from build123d import *

# Parameters (mm, degrees)
SKETCH_1_W          = 390
SKETCH_1_H          = 70
EXTRUDE_1_DEPTH     = 90
SKETCH_2_W          = 20
SKETCH_2_H          = 20
CUT_EXTRUDE_1_DEPTH = 85
CUT_EXTRUDE_2_DEPTH = 20
CUT_EXTRUDE_3_DEPTH = 20
CUT_EXTRUDE_4_DEPTH = 86.5


with BuildPart() as part:
    # 草圖1 → 填料-伸長1 (new body)
    with BuildSketch(Plane(origin=(0, 0, 0), x_dir=(1, 0, 0), z_dir=(0, 1, 0))):
        Rectangle(SKETCH_1_W, SKETCH_1_H)
    extrude(amount=EXTRUDE_1_DEPTH)

    # 草圖2 → 除料-伸長1 (cut)
    with BuildSketch(Plane.XY.offset(35)):
        with Locations((185, 10)):
            Rectangle(SKETCH_2_W, SKETCH_2_H)
        with Locations((-185, 10)):
            Rectangle(SKETCH_2_W, SKETCH_2_H)
    extrude(amount=-CUT_EXTRUDE_1_DEPTH, mode=Mode.SUBTRACT)

    # 草圖3 → 除料-伸長2 (cut)
    with BuildSketch(Plane(origin=(195, 0, 0), x_dir=(0, 0, -1), z_dir=(1, 0, 0))):
        Polygon((35, 20), (11.5, 20), (35, 43.5), align=None)
    cut_extrude_2 = extrude(amount=-CUT_EXTRUDE_2_DEPTH, mode=Mode.SUBTRACT)

    # 鏡射1: 除料-伸長2 across plane
    add(cut_extrude_2.mirror(Plane(origin=(0, 0, 0), x_dir=(0, 0, 1), z_dir=(1, 0, 0))), mode=Mode.SUBTRACT)

    # 草圖4 → 除料-伸長3 (cut)
    with BuildSketch(Plane.XZ):
        Polygon((-151.5, -35), (-175, -35), (-175, -11.5), align=None)
        Polygon((175, -11.5), (151.5, -35), (175, -35), align=None)
    extrude(amount=-CUT_EXTRUDE_3_DEPTH, mode=Mode.SUBTRACT)

    # 草圖5 → 除料-伸長4 (cut)
    with BuildSketch(Plane(origin=(0, 90, 0), x_dir=(1, 0, 0), z_dir=(0, 1, 0))):
        Polygon((-171.5, 10.050252532), (-171.5, -31.5), (171.5, -31.5), (171.5, 10.050252532), (150.050252532, 31.5), (-150.050252532, 31.5), align=None)
    extrude(amount=-CUT_EXTRUDE_4_DEPTH, mode=Mode.SUBTRACT)


solid = part.part
Verification items for the finished model (mm, model axes). A direction names the side the tool comes from. Coordinates: 2 decimals unless noted, no trailing zeros. Order: outer loops, then holes, each group sorted by start corner. A loop starts at its lowest first (then second) coordinate and runs counter-clockwise, first axis right, second up.
Item 1: Section check D-D, the plane y = 48.5. Enter the section's corners in (x, z), then the cut area to 3 significant figures.
Filled in:
outline: (-195, -35) - (195, -35) - (195, 35) - (-195, 35) - close; hole (-171.5, -10.05) - (-150.05, -31.5) - (150.05, -31.5) - (171.5, -10.05) - (171.5, 31.5) - (-171.5, 31.5) - close
area: 6,150 mm2
Item 2: Section check C-C, the plane x = 134. Enter the section's corners in (y, z), then the cut area to 4 significant figures.
Filled in:
outline: (0, -35) - (90, -35) - (90, -31.5) - (3.5, -31.5) - (3.5, 31.5) - (90, 31.5) - (90, 35) - (0, 35) - close
area: 850.5 mm2
Item 3: Depth check by flat-ended pin: pin 1 (12 mm diameter, centred on x = 76.5, z = 23.5, fed in from +Y); pin 2 (22 mm diameter, centred on x = 187, z = 16.5, fed in from -Y); pin 3 (1.5 mm diameter, centred on y = 21.5, z = -18, fed in from +X). Enter the tip coordinate at first touch or a pass-through.
Filled in:
pin 1: stops at y = 3.5
pin 2: stops at y = 20
pin 3: stops at x = 175
Item 4: Section check B-B, the plane z = -3. Enter the section's corners in (x, y).
Filled in:
outline: (-195, 20) - (-175, 20) - (-175, 0) - (175, 0) - (175, 20) - (195, 20) - (195, 90) - (171.5, 90) - (171.5, 3.5) - (-171.5, 3.5) - (-171.5, 90) - (-195, 90) - close
Item 5: Section check A-A, the plane y = 27. Enter the section's corners in (x, z).
Filled in:
outline: (-195, -18.5) - (-175, -18.5) - (-175, -35) - (175, -35) - (175, -18.5) - (195, -18.5) - (195, 35) - (-195, 35) - close; hole (-171.5, -10.05) - (-150.05, -31.5) - (150.05, -31.5) - (171.5, -10.05) - (171.5, 31.5) - (-171.5, 31.5) - close
Item 6: Access from +Z, -Z, +X, -X, +Y, -Y to the whole of each face (thin tool, end or side, straight path). Record for faces 4 (the face through (185.1, 31.6, -23.1)), 5 (the face through (-185.1, 31.6, -23.1)), 6 (the face through (185, 20, 12)), 7 (the face through (-2, 47, 31.5)).
Filled in:
face 4: -Z, +X, -Y
face 5: -Z, -X, -Y
face 6: +Z, -Z, +X, -Y
face 7: +Y
Item 7: Material ranges on L1, parallel to Z at x = -140.5, y = 5.5; L2, parallel to X at y = 17.5, z = 14.5; L3, parallel to X at y = 47, z = 1, recorded low to high.
Filled in:
L1: z = -35 to -31.5, 31.5 to 35
L2: x = -175 to -171.5, 171.5 to 175
L3: x = -195 to -171.5, 171.5 to 195
Item 8: Release check for a two-part mould opening along Z. For faces 1 (the face through (-171.5, 47, 10)), 2 (the face through (175, 10, 12)), 3 (the face through (-3, 44, 35)) record: +Z half, -Z half, draft (parallel to the pull), parting line (faces both ways), or undercut.
Filled in:
face 1: undercut
face 2: draft
face 3: +Z half
